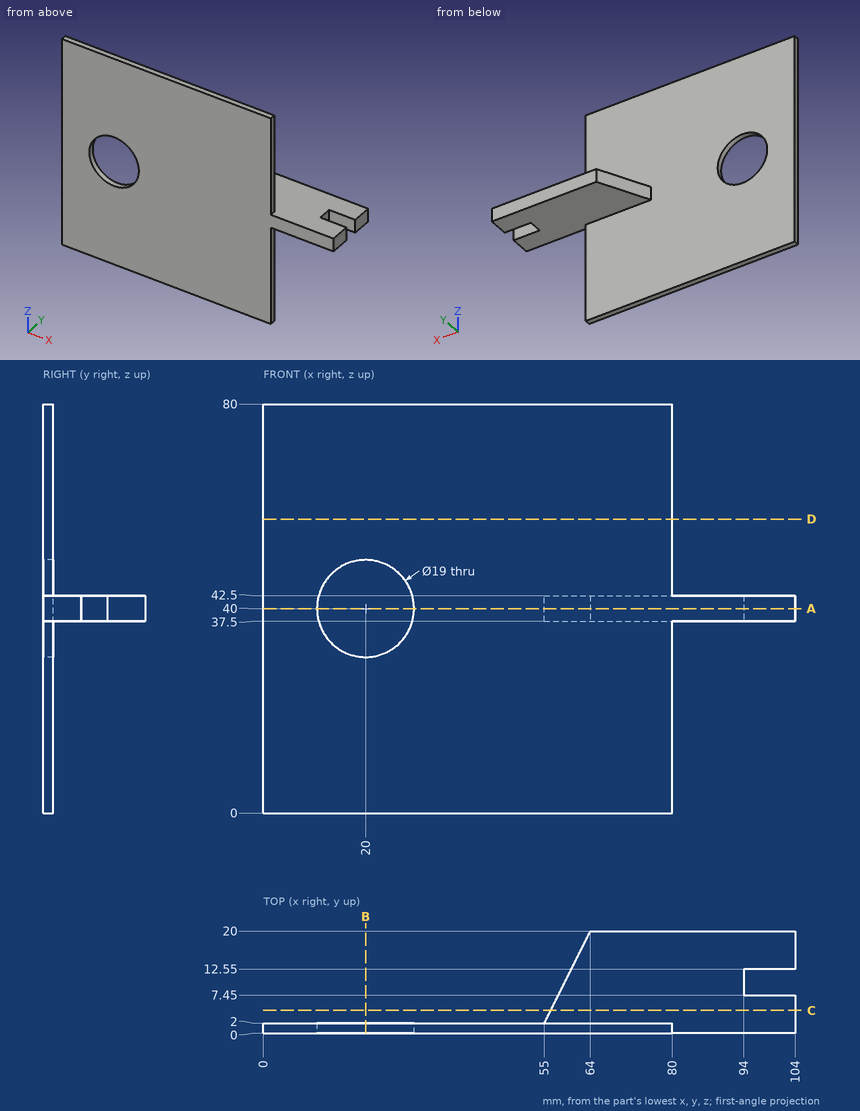
Part print with two shaded views. Sizes in mm from the minimum x, y, z corner. Round coordinates to 2 decimals unless told otherwise and drop trailing zeros. Order: outer loops, then holes, each group sorted by start corner. A loop starts at its lowest first (then second) coordinate and runs counter-clockwise, first axis right, second up.
(1) Band-saw the part on A-A (z = 40). List the corners of the cut face in (x, y), then the cut area to 3 significant figures.
(2) Pin check, flat tips, straight feed: pin 1 (0.6 mm diameter, centred on y = 1, z = 26.5, fed in from +X); pin 2 (1 mm diameter, centred on x = 71.5, z = 13, fed in from +Y); pin 3 (6 mm diameter, centred on x = 69.5, y = 15.5, fed in from -Z). Stop position of each tip, or through.
(3) Band-saw the part on B-B (x = 20). List the corners of the cut face in (y, z).
(4) Drill centre lines: line 1 (Z direction, x = 20, y = 1.45); line 2 (Y direction, x = 24, z = 69); line 3 (Z direction, x = 98, y = 4). Where is each one in solid material? Low to high.
(5) Band-saw the part on C-C (y = 4.5). List the corners of the cut face in (x, z), then the cut area to 3 significant figures.
(6) Band-saw the part on D-D (z = 57.5). List the corners of the cut face in (x, y).
Verdict:
1. outline: (0, 0) - (10.5, 0) - (10.5, 2) - (0, 2) - close; (29.5, 0) - (104, 0) - (104, 7.45) - (94, 7.45) - (94, 12.55) - (104, 12.55) - (104, 20) - (64, 20) - (55, 2) - (29.5, 2) - close
1. area: 920 mm2
2. pin 1: stops at x = 80
2. pin 2: stops at y = 2
2. pin 3: stops at z = 37.5
3. outline: (0, 0) - (2, 0) - (2, 30.5) - (0, 30.5) - close; (0, 49.5) - (2, 49.5) - (2, 80) - (0, 80) - close
4. line 1: z = 0 to 30.5, 49.5 to 80
4. line 2: y = 0 to 2
4. line 3: z = 37.5 to 42.5
5. outline: (56.25, 37.5) - (104, 37.5) - (104, 42.5) - (56.25, 42.5) - close
5. area: 239 mm2
6. outline: (0, 0) - (80, 0) - (80, 2) - (0, 2) - close
